Autodesk Fusion 360 part; units mm, degrees
sketch "Sketch1" plane through (0, 0, 0) normal (0, 0, 1) x (1, 0, 0)
  line L0 (-135, 128.4755) -> (-30.225, 128.4755)
  line L1 (-30.225, 128.4755) -> (-30.225, 60.0051)
  line L2 (-30.225, 60.0051) -> (-135, 60.0051)
  line L3 (-135, 60.0051) -> (-135, 128.4755)
  circle A0 centre (-34.9919, 122.4579) radius 0.7
  circle A1 centre (-125.5089, 122.4579) radius 0.7
  circle A2 centre (-140, 135) radius 3
  circle A3 centre (-25, 135) radius 3
  circle A4 centre (-25, 50) radius 3
  circle A5 centre (-140, 50) radius 3
  line L4 (-145, 140) -> (-20, 140)
  line L5 (-20, 140) -> (-20, 45)
  line L6 (-20, 45) -> (-145, 45)
  line L7 (-145, 45) -> (-145, 140)
  circle A6 centre (-25, 135) radius 1.7
  circle A7 centre (-140, 135) radius 1.7
  circle A8 centre (-140, 50) radius 1.7
  circle A9 centre (-25, 50) radius 1.7
  dimension "d1" = 104.775
  dimension "d2" = 68.4704
  dimension "d17" = 1.4
  dimension "d18" = 1.4
  dimension "d24" = 6
  dimension "d25" = 6
  dimension "d26" = 6
  dimension "d28" = 6
  dimension "d29" = 3.4
  dimension "d30" = 3.4
  dimension "d31" = 3.4
  dimension "d32" = 3.4
extrude "Extrude1" add sketch "Sketch1" along normal blind 9.9 from surface at 3.1 contours A2 | A3 | A4 | A5 makes body 1 at (-22.2356, 136.1653, 9.7) makes body 2 at (-137.2356, 136.1653, 9.7) makes body 3 at (-22.0037, 49.8505, 9.7) makes body 4 at (-139.1875, 52.8879, 9.7)
extrude "Extrude2" add sketch "Sketch1" along normal blind 13 contours L4 L5 L6 L7 bodies 1 2 3 4
extrude "Extrude3" add sketch "Sketch1" along normal blind 3 contours L0 L1 L2 L3 bodies 1
extrude "Extrude4" add sketch "Sketch1" along normal blind 8 contours A0 | A1 bodies 1
sketch "Sketch2" plane through (0, 0, 13) normal (0, 0, 1) x (-1, 0, 0)
  circle A0 centre (25, -135) radius 1.7
  circle A1 centre (140, -50) radius 1.7
  line L0 (30.225, -60.0051) -> (135, -60.0051)
  line L1 (135, -60.0051) -> (135, -128.4755)
  line L2 (135, -128.4755) -> (30.225, -128.4755)
  line L3 (30.225, -128.4755) -> (30.225, -60.0051)
  line L4 (145, -45) -> (20, -45)
  line L5 (20, -45) -> (20, -140)
  line L6 (20, -140) -> (145, -140)
  line L7 (145, -140) -> (145, -45)
  circle A2 centre (140, -135) radius 1.7
  circle A3 centre (25, -50) radius 1.7
  line L8 (94.9004, -128.4755) -> (94.9004, -140)
  line L9 (70, -140) -> (70, -128.4755)
extrude "Extrude5" cut sketch "Sketch2" against normal blind 7.5 contours L2 L6 L8 L9 bodies 1
fillet "Fillet1" radius 5 4 edges at (-145, 45, 6.5) (-145, 140, 6.5) (-20, 140, 6.5) (-20, 45, 6.5) on bodies 1
fillet "Fillet2" radius 2.5 8 edges at (-143.5355, 138.5355, 0) (-82.5, 140, 0) (-21.4645, 138.5355, 0) (-20, 92.5, 0) (-21.4645, 46.4645, 0) (-82.5, 45, 0) (-143.5355, 46.4645, 0) (-145, 92.5, 0) on bodies 1
extrude "Extrude6" add sketch "Sketch1" along normal blind 2 contours A2 | A3 | A4 | A5 | A6 | A7 | A8 | A9 bodies 1
extrude "Extrude7" cut sketch "Sketch1" along normal blind 1 contours A2 | A3 | A4 | A5 | A6 | A7 | A8 | A9 bodies 1
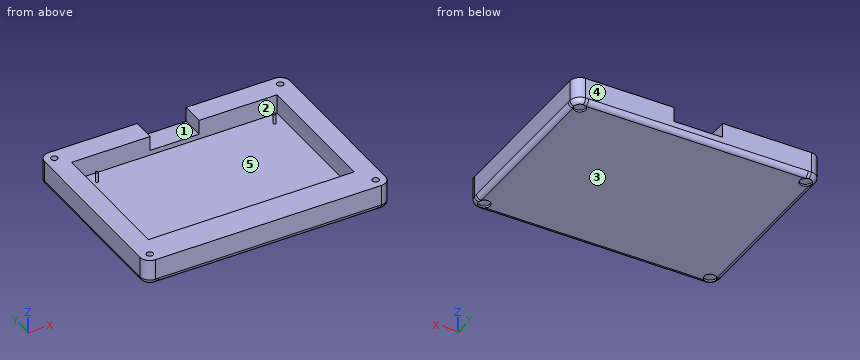
CAD build for the part. Positions are in the model's coordinates, mm. Face numbers are marked on the shaded views. A direction names the side the tool comes from. Round coordinates to 2 decimals unless told otherwise and drop trailing zeros. Loops run counter-clockwise (first coordinate to the right, second up) from the corner with the lowest first, then second, coordinate; pieces in that order, holes last. Notation, with made-up numbers: (34.25, 63.5) - (56.25, 63.5) arc R24 cw to (56.25, 75.5) - close; hole circle Ø4 at (44, 41). An arc over 180 degrees is marked (long way). Return JSON: item names as keys, results as strings. Group by question number.
Q1. Drill centre lines: line 1 along Y through (x, z) = (-140, 9.5); line 2 along Y through (x, z) = (-25, 2.3); line 3 along X through (y, z) = (135, 6.25). Where is each one in solid material? Low to high. Write a range as [from, to].
Q2. Tool access for the marked faces 1, 2 and 3: list every direction of +Z, -Z, +X, -X, +Y, -Y with a clear straight run to the whole face (end or side of a thin tool).
Q3. Band-saw the part on B-B on y = 113.5. Give the cut face in (x, z) (3 decimals).
Q4. Band-saw the part on A-A on z = 9.5. Give the cut face in (x, y) (1 decimal).
Q5. Two-plate mould, pull along X, no slides. Class the marked faces 4 and 5: +X half, -X half, draft (parallel to the pull), parting line (faces both ways), or undercut.
Q6. Flat gauge pins, fed straight in: pin 1 Ø1.8 at (x, y) = (-138.5, 135) entering from -Z; pin 2 Ø6 at (x, y) = (-46, 106.5) entering from +Z. Where does each tip first touch, or does it go through?
Solutions:
{
 "1": {"line 1": "y = [45, 48.3], [51.7, 133.3], [136.7, 140]", "line 2": "y = [45, 47], [53, 132], [138, 140]", "line 3": "x = [-145, -141.7], [-138.3, -94.9], [-70, -26.7], [-23.3, -20]"},
 "2": {"face 1": "+Z, +Y", "face 2": "+Z", "face 3": "-Z, +X, -X, +Y, -Y"},
 "3": {"outline": "(-145, 2.5) arc R2.5 ccw to (-142.5, 0) - (-22.5, 0) arc R2.5 ccw to (-20, 2.5) - (-20, 13) - (-30.225, 13) - (-30.225, 3) - (-135, 3) - (-135, 13) - (-145, 13) - close"},
 "4": {"outline": "(-145, 50) arc R5 ccw to (-140, 45) - (-25, 45) arc R5 ccw to (-20, 50) - (-20, 135) arc R5 ccw to (-25, 140) - (-70, 140) - (-70, 128.5) - (-30.2, 128.5) - (-30.2, 60) - (-135, 60) - (-135, 128.5) - (-94.9, 128.5) - (-94.9, 140) - (-140, 140) arc R5 ccw to (-145, 135) - close; hole circle Ø3.4 at (-140, 50); hole circle Ø3.4 at (-140, 135); hole circle Ø3.4 at (-25, 50); hole circle Ø3.4 at (-25, 135)"},
 "5": {"face 4": "draft", "face 5": "undercut"},
 "6": {"pin 1": "stops at z = 1", "pin 2": "stops at z = 3"}
}
